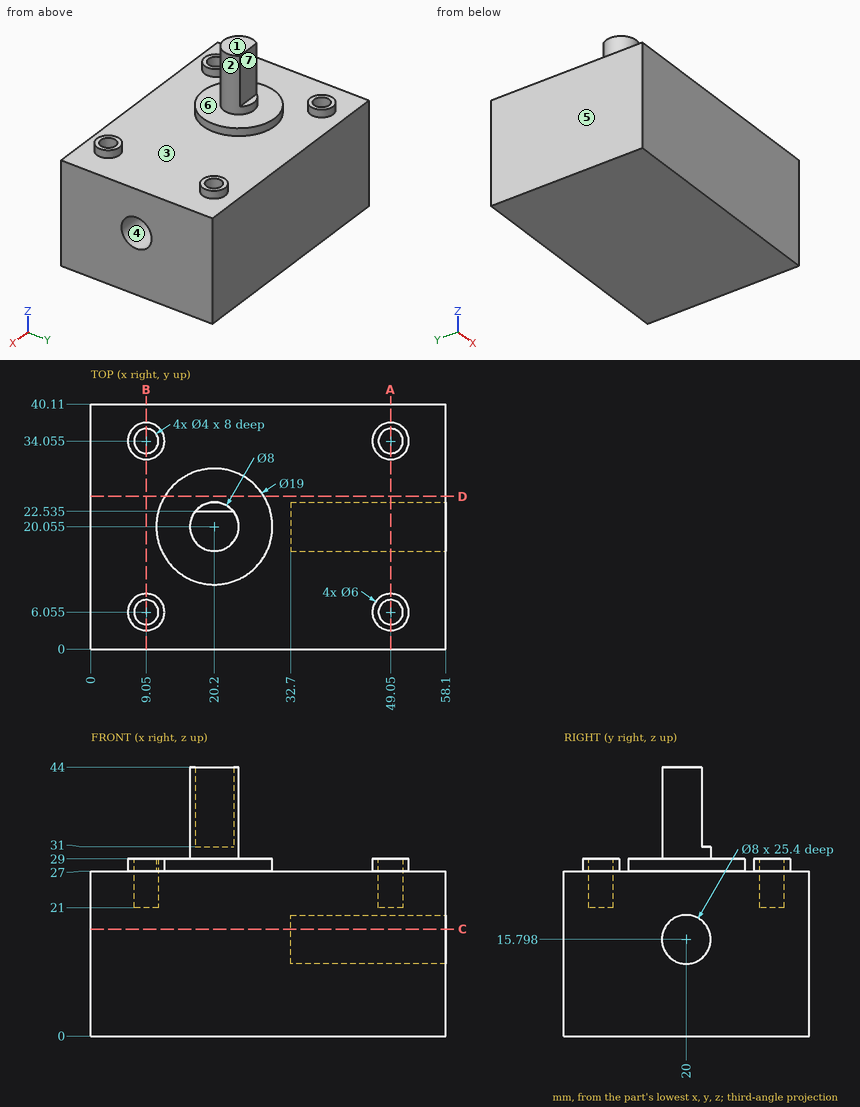
Study the drawing (mm; zero at the part's minimum x, y, z) and answer. A direction names the side the tool comes from. Coordinates: 2 decimals unless noted, no trailing zeros. Order: outer loops, then holes, each group sorted by start corner. A loop starts at its lowest first (then second) coordinate and runs counter-clockwise, first axis right, second up. Notation, with made-up numbers: (17.25, 4.5) -> (56.25, 4.5) arc R21 cw to (56.25, 36.5) -> close; hole circle Ø4 at (-20, 54). An arc over 180 degrees is marked (long way). Answer in a Markdown table with one row per item. Add a question column.
Item 1: Find section C-C (z = 17.5). Write down the section's boundary in (x, y), then the cut area to 3 significant figures.
Item 2: Determine the mould class of the marked faces 1, 2 and 3 for opening direction Y: +Y half, -Y half, draft (parallel to the pull), parting line (faces both ways), or undercut.
Item 3: Each of these flat-tipped pins is pushed along its axis until it touches: P1, Ø5, axis at x = 50, y = 7, coming from the +Z side; P2, Ø4, axis at y = 19.5, z = 16, coming from the +X side; P3, Ø2, axis at x = 21.5, z = 39.5, coming from the -Y side; P4, Ø8, axis at x = 32, z = 34, coming from the +Y side. Where does it stop, or does it pass through?
Item 4: Find section D-D (y = 25). Write down the section's boundary in (x, z).
Item 5: Which of the six approach directions +Z, -Z, +X, -X, +Y, -Y give full straight-line access (tool end or side, diameter ignored) to the marked faces 4, 5, 6 and 7?
Item 6: Find section A-A (x = 49.05). Write down the section's boundary in (y, z) (3 decimals).
Item 7: Find section B-B (x = 9.05). Write down the section's boundary in (y, z) (3 decimals), then the cut area to 3 significant figures.
Item 8: Find the intervals of material crossed by L1, parallel to Y at x = 49.05, z = 23.25 (3 decimals); L2, parallel to Z at x = 29.5, y = 10; L3, parallel to Z at x = 13.5, y = 15.5, in increasing order. Write a range as from..to.
Result set:
| question | item | result |
|---|---|---|
| 1 | outline | (0, 0) -> (58.1, 0) -> (58.1, 16.38) -> (32.7, 16.38) -> (32.7, 23.62) -> (58.1, 23.62) -> (58.1, 40.11) -> (0, 40.11) -> close |
| 1 | area | 2,150 mm² |
| 2 | face 1 | draft |
| 2 | face 2 | parting line |
| 2 | face 3 | undercut |
| 3 | P1 | stops at z = 29 |
| 3 | P2 | stops at x = 32.7 |
| 3 | P3 | stops at y = 16.07 |
| 3 | P4 | passes through |
| 4 | outline | (0, 0) -> (58.1, 0) -> (58.1, 27) -> (28.31, 27) -> (28.31, 29) -> (12.09, 29) -> (12.09, 27) -> (0, 27) -> close |
| 5 | face 4 | +X |
| 5 | face 5 | +Z, -Z, -X, +Y, -Y |
| 5 | face 6 | +Z |
| 5 | face 7 | +Z, +X, -X, +Y |
| 6 | outline | (0, 0) -> (40.11, 0) -> (40.11, 27) -> (37.055, 27) -> (37.055, 29) -> (36.055, 29) -> (36.055, 21) -> (32.055, 21) -> (32.055, 29) -> (31.055, 29) -> (31.055, 27) -> (9.055, 27) -> (9.055, 29) -> (8.055, 29) -> (8.055, 21) -> (4.055, 21) -> (4.055, 29) -> (3.055, 29) -> (3.055, 27) -> (0, 27) -> close; hole circle Ø8 at (20, 15.798) |
| 7 | outline | (0, 0) -> (40.11, 0) -> (40.11, 27) -> (37.055, 27) -> (37.055, 29) -> (36.055, 29) -> (36.055, 21) -> (32.055, 21) -> (32.055, 29) -> (31.055, 29) -> (31.055, 27) -> (9.055, 27) -> (9.055, 29) -> (8.055, 29) -> (8.055, 21) -> (4.055, 21) -> (4.055, 29) -> (3.055, 29) -> (3.055, 27) -> (0, 27) -> close |
| 7 | area | 1,040 mm² |
| 8 | L1 | y = 0..4.055, 8.055..32.055, 36.055..40.11 |
| 8 | L2 | z = 0..27 |
| 8 | L3 | z = 0..29 |
